Source: three-view drawing plus pictorial views. Frame: mm from the lowest corner of the part. A direction names the side the tool comes from. Give positions to 0.01 mm unless a question says otherwise; leave off trailing zeros. Loops run counter-clockwise (first coordinate to the right, second up) from the corner with the lowest first, then second, coordinate; pieces in that order, holes last.
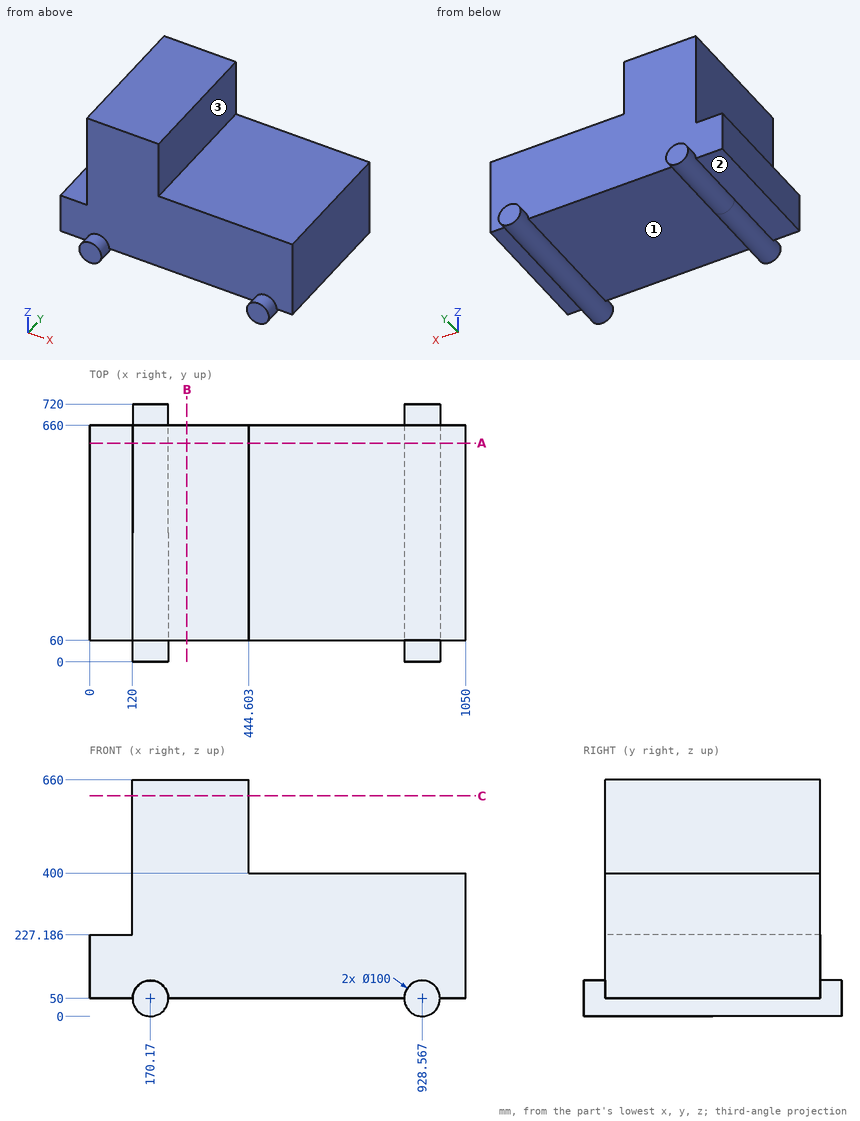
Q1. Material intervals for probe 1 along Y at (x, z) = (323, 525.5); probe 2 along X at (y, z) = (398, 475); probe 3 along X at (y, z) = (122, 299), sorted ascending.
Q2. Section query C-C, the plane z = 615.5. Return loops of the section in (x, y).
Q3. Section query B-B, the plane x = 271.5. Return loops of the section in (y, z).
Q4. Section query A-A, the plane y = 611. Return loops of the section in (x, z).
Q5. Reachability of the marked faces 1, 2 and 3 from +Z, -Z, +X, -X, +Y, -Y: full face, straight path, thin tool, end or side. Return the list, or none.
Q6. Pin query (flat end, axial travel): pin 1 Ø4 at (x, z) = (205.5, 346.5) entering from -Y; pin 2 Ø10 at (y, z) = (543, 254) entering from -X; pin 3 Ø1.5 at (x, y) = (847, 552.5) entering from +Z. Return the tip coordinate at first contact, or that it passes through.
Resolved:
1. probe 1: y = 60 to 660
1. probe 2: x = 120 to 444.6
1. probe 3: x = 120 to 1050
2. outline: (120, 60) - (444.6, 60) - (444.6, 660) - (120, 660) - close
3. outline: (60, 50) - (660, 50) - (660, 660) - (60, 660) - close
4. outline: (0, 50) - (120.17, 50) arc R50 ccw to (220.17, 50) - (878.57, 50) arc R50 ccw to (978.57, 50) - (1050, 50) - (1050, 400) - (444.6, 400) - (444.6, 660) - (120, 660) - (120, 227.19) - (0, 227.19) - close
5. face 1: -Z, +Y, -Y
5. face 2: -Z, -X, +Y, -Y
5. face 3: +Z, +X, +Y, -Y
6. pin 1: stops at y = 60
6. pin 2: stops at x = 120
6. pin 3: stops at z = 400
